The model under review builds one solid part; all positions refer to its coordinate system, in mm. A direction names the side the tool comes from. Give positions to 0.01 mm unless a question says otherwise; leave off trailing zeros. Loops run counter-clockwise (first coordinate to the right, second up) from the corner with the lowest first, then second, coordinate; pieces in that order, holes last. Notation, with made-up numbers: M 78.5,46 L 131.5,46 A28 ccw 131.5,82 Z; hole C 41.25,42 d3. An arc over 180 degrees is marked long. Return JSON: item names as keys, results as strings.
```python
from build123d import *

# Parameters (mm, degrees)
F2_DEPTH = 3.2
F3_DEPTH = 3.15


with BuildPart() as f2:
    # F1 (on Front) → F2 (new body, symmetric)
    with BuildSketch(Plane.XZ):
        with BuildLine():
            Line((12, 6.3), (12, 0))
            Line((12, 0), (-12, 0))
            Line((-12, 0), (-12, 6.3))
            Line((-12, 6.3), (-15, 6.3))
            Line((-15, 6.3), (-15, 12.8))
            Line((-15, 12.8), (-20, 12.8))
            ThreePointArc((-20, 12.8), (-23.5199404292, 5.9790524317), (-24.7337240148, -1.6))
            Line((-24.7337240148, -1.6), (-24.7337240148, -2.8))
            ThreePointArc((-24.7337240148, -2.8), (-23.0543551323, -6.8543551323), (-19, -8.5337240148))
            Line((-19, -8.5337240148), (-7.6, -8.5337240148))
            ThreePointArc((-7.6, -8.5337240148), (-6.705572809, -8.3225783968), (-6, -7.7337240148))
            Line((-6, -7.7337240148), (6, -7.7337240148))
            ThreePointArc((6, -7.7337240148), (6.705572809, -8.3225783968), (7.6, -8.5337240148))
            Line((7.6, -8.5337240148), (19, -8.5337240148))
            ThreePointArc((19, -8.5337240148), (23.0543551323, -6.8543551323), (24.7337240148, -2.8))
            Line((24.7337240148, -2.8), (24.7337240148, -1.6))
            ThreePointArc((24.7337240148, -1.6), (23.5199404292, 5.9790524317), (20, 12.8))
            Line((20, 12.8), (15, 12.8))
            Line((15, 12.8), (15, 6.3))
            Line((15, 6.3), (12, 6.3))
        make_face()
    extrude(amount=F2_DEPTH, both=True)

    # F1 (on Front) → F3 (join, symmetric)
    with BuildSketch(Plane.XZ):
        with BuildLine():
            add(Edge.make_bspline(
                [(16.5, 19.2), (14.5000000527, 19.2), (13.7500000527, 16), (13.0000000527, 12.8), (15, 12.8)],
                knots=[0.2076781727, 0.2076781727, 0.2076781727, 1.7784744995, 1.7784744995, 3.3492708263, 3.3492708263, 3.3492708263], degree=2, weights=[1, 0.7071067812, 1, 0.7071067812, 1]))
            Line((15, 12.8), (20, 12.8))
            ThreePointArc((20, 12.8), (23.5199404292, 5.9790524317), (24.7337240148, -1.6))
            Line((24.7337240148, -1.6), (24.7337240148, -2.8))
            ThreePointArc((24.7337240148, -2.8), (23.0543551323, -6.8543551323), (19, -8.5337240148))
            Line((19, -8.5337240148), (7.6, -8.5337240148))
            ThreePointArc((7.6, -8.5337240148), (6.705572809, -8.3225783968), (6, -7.7337240148))
            Line((6, -7.7337240148), (-6, -7.7337240148))
            ThreePointArc((-6, -7.7337240148), (-6.705572809, -8.3225783968), (-7.6, -8.5337240148))
            Line((-7.6, -8.5337240148), (-19, -8.5337240148))
            ThreePointArc((-19, -8.5337240148), (-23.0543551323, -6.8543551323), (-24.7337240148, -2.8))
            Line((-24.7337240148, -2.8), (-24.7337240148, -1.6))
            ThreePointArc((-24.7337240148, -1.6), (-23.5199404292, 5.9790524317), (-20, 12.8))
            Line((-20, 12.8), (-15, 12.8))
            add(Edge.make_bspline(
                [(-14.9999999473, 12.8), (-13, 12.8), (-13.7499999802, 15.9999999157), (-14.4999999605, 19.1999998315), (-16.4999999473, 19.2)],
                knots=[6.0755071131, 6.0755071131, 6.0755071131, 7.6463034136, 7.6463034136, 9.217099714, 9.217099714, 9.217099714], degree=2, weights=[1, 0.7071067905, 1, 0.7071067905, 1]))
            Line((-16.5, 19.2), (-20, 19.2))
            ThreePointArc((-20, 19.2), (-26.653524819, 9.7318136236), (-29, -1.6))
            Line((-29, -1.6), (-29, -2.8))
            ThreePointArc((-29, -2.8), (-26.0710678119, -9.8710678119), (-19, -12.8))
            Line((-19, -12.8), (19, -12.8))
            ThreePointArc((19, -12.8), (26.0710678119, -9.8710678119), (29, -2.8))
            Line((29, -2.8), (29, -1.6))
            ThreePointArc((29, -1.6), (26.653524819, 9.7318136236), (20, 19.2))
            Line((20, 19.2), (16.5, 19.2))
        make_face()
    extrude(amount=F3_DEPTH, both=True)


solid = f2.part
```
1) The part is to be moulded in two halves that separate along X. For faces 1 (the face through (-26.59, -0.04, 9.88)), 2 (the face through (-12, 0, 3)), 3 (the face through (0, -3.2, -2)), say which applies: released by +X, released by -X, zero draft, split by the parting line, or undercut.
From the geometry:
{"face 1": "released by -X", "face 2": "undercut", "face 3": "zero draft"}
2) Wall thickness on L1, parallel to Z at x = -8, y = 2.5; L2, parallel to X at y = -2.25, z = -11; L3, parallel to Z at x = 14.5, y = 3: over which ranges is each line inside the solid? List them lowest first. Write a range as from..to.
From the geometry:
{"L1": "-12.8..0", "L2": "-24.72..24.72", "L3": "-12.8..6.3, 12.91..17.77"}
3) Consider section C-C on z = 11.5. Write out the cut boundary in (x, y).
From the geometry:
{"outline": "M -25.82,-3.15 L -20.89,-3.15 L -20.89,-3.2 L -15,-3.2 L -15,3.2 L -20.89,3.2 L -20.89,3.15 L -25.82,3.15 Z; M 15,-3.2 L 20.89,-3.2 L 20.89,-3.15 L 25.82,-3.15 L 25.82,3.15 L 20.89,3.15 L 20.89,3.2 L 15,3.2 Z"}
4) Consider section B-B on x = 1.5. Write out the cut boundary in (y, z).
From the geometry:
{"outline": "M -3.2,-7.73 L -3.15,-7.73 L -3.15,-12.8 L 3.15,-12.8 L 3.15,-7.73 L 3.2,-7.73 L 3.2,0 L -3.2,0 Z"}
5) Consider section A-A on z = 7. Write out the cut boundary in (x, y).
From the geometry:
{"outline": "M -27.67,-3.15 L -23.16,-3.15 L -23.16,-3.2 L -15,-3.2 L -15,3.2 L -23.16,3.2 L -23.16,3.15 L -27.67,3.15 Z; M 15,-3.2 L 23.16,-3.2 L 23.16,-3.15 L 27.67,-3.15 L 27.67,3.15 L 23.16,3.15 L 23.16,3.2 L 15,3.2 Z"}
6) Consider section D-D on x = 10. Write out the cut boundary in (y, z).
From the geometry:
{"outline": "M -3.2,-8.53 L -3.15,-8.53 L -3.15,-12.8 L 3.15,-12.8 L 3.15,-8.53 L 3.2,-8.53 L 3.2,0 L -3.2,0 Z"}
7) Insertion check: pin 1 (3.5 mm diameter, centred on x = -14, y = 0, fed in from +Z); pin 2 (1.9 mm diameter, centred on y = -1, z = 8.5, fed in from +X); pin 3 (2 mm diameter, centred on x = 12, y = -2, fed in from +Z). Each pin has a flat end and moves straight along its axis. Give the tip position at first contact, or say it passes through.
From the geometry:
{"pin 1": "z = 19", "pin 2": "x = 27.49", "pin 3": "z = 6.3"}
8) Tool access review of faces 4 (the face through (15, 0, 10)), 5 (the face through (2, 3.15, -9)), 6 (the face through (12, 0, 3)): name each direction out of +Z, -Z, +X, -X, +Y, -Y from which nothing blocks a thin tool from reaching the whole face with its end or side.
From the geometry:
{"face 4": "+Y, -Y", "face 5": "+Y", "face 6": "+Z, +Y, -Y"}
